```python
from build123d import *

# Parameters (mm, degrees)
SKETCH1_W           = 6
SKETCH1_H           = 60
SKETCH1_R           = 1.5
BOSS_EXTRUDE1_DEPTH = 2


with BuildPart() as part:
    # Sketch1 → Boss-Extrude1 (new body)
    with BuildSketch(Plane(origin=(0, 0, 0), x_dir=(1, 0, 0), z_dir=(0, 1, 0))):
        Rectangle(SKETCH1_W, SKETCH1_H)
        with Locations((0, -20)):
            Circle(SKETCH1_R, mode=Mode.SUBTRACT)
        with Locations((0, 20)):
            Circle(SKETCH1_R, mode=Mode.SUBTRACT)
        with BuildLine():
            Line((-3, -30), (3, -30))
            ThreePointArc((3, -30), (0, -33), (-3, -30))
        make_face()
        with BuildLine():
            ThreePointArc((-3, 30), (0, 33), (3, 30))
            Line((3, 30), (-3, 30))
        make_face()
    extrude(amount=BOSS_EXTRUDE1_DEPTH)


solid = part.part
```
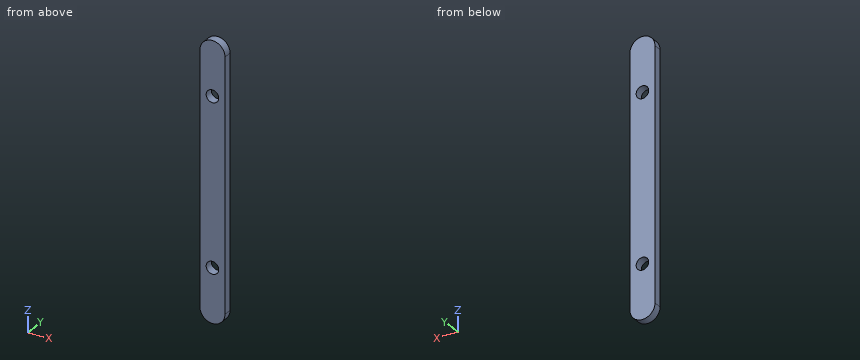
Verification items for the finished model (mm, model axes). Coordinates: 2 decimals unless noted, no trailing zeros. Write each loop counter-clockwise with the first axis right and the second up, starting at its lowest first coordinate (ties: lowest second). Pieces come first, ordered by that corner, then holes. Notation, with made-up numbers: (-14.5, 17.5) - (20.5, 17.5) arc R22 cw to (20.5, 39.5) - close; hole circle Ø7 at (69, 84.5). An arc over 180 degrees is marked (long way). One line per question, with ' | ' between items. Start each with the question number.
1. Section check A-A (z = 20). Enter the section's corners in (x, y), plus the area to 3 significant figures.
2. Material ranges on line 1 along Z through (x, y) = (0, 0.75); line 2 along X through (y, z) = (0.9, 20); line 3 along Z through (x, y) = (1.2, 0.7), recorded low to high.
3. Section check C-C (y = 0.6). Enter the section's corners in (x, z).
4. Gauge pin test, flat end, axial feed: P1, Ø3, axis at x = 0.5, z = -17, coming from the -Y side. Record the tip position at first contact, or that the pin passes through.
5. Section check B-B (x = 0). Enter the section's corners in (y, z), plus the area to 3 significant figures.
Computed values:
1) outline: (-3, 0) - (-1.5, 0) - (-1.5, 2) - (-3, 2) - close; (1.5, 0) - (3, 0) - (3, 2) - (1.5, 2) - close | area: 6.00 mm²
2) line 1: -33 to -21.5, -18.5 to 18.5, 21.5 to 33 | line 2: -3 to -1.5, 1.5 to 3 | line 3: -32.75 to -20.9, -19.1 to 19.1, 20.9 to 32.75
3) outline: (-3, -30) arc R3 ccw to (3, -30) - (3, 30) arc R3 ccw to (-3, 30) - close; hole circle Ø3 at (0, -20); hole circle Ø3 at (0, 20)
4) P1: y = 0
5) outline: (0, -33) - (2, -33) - (2, -21.5) - (0, -21.5) - close; (0, -18.5) - (2, -18.5) - (2, 18.5) - (0, 18.5) - close; (0, 21.5) - (2, 21.5) - (2, 33) - (0, 33) - close | area: 120 mm²
